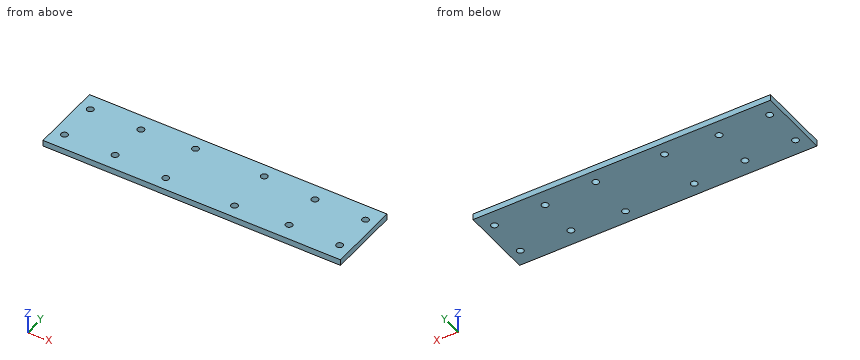
from build123d import *

# Parameters (mm, degrees)
SKETCH_1_W                  = 147
SKETCH_1_H                  = 36
EXTRUDE_1_DEPTH             = 3
HOLE_WIZARD_M4_2_AT_2_COUNT = 2
HOLE_WIZARD_M4_2_AT_2_PITCH = 25


with BuildPart() as part:
    # 草图1 → 凸台-拉伸1 (new body)
    with BuildSketch(Plane.XY):
        Rectangle(SKETCH_1_W, SKETCH_1_H)
    extrude(amount=EXTRUDE_1_DEPTH)

    # 草图3 → M4 螺纹孔的螺纹孔钻头1 (revolve, cut)
    with BuildSketch(Plane(origin=(-17, 11.5, 3), x_dir=(0, -1, 0), z_dir=(1, 0, 0))):
        Polygon((0, 0), (0, 10.991420021), (1.65, 10), (1.65, 0), align=None)
    hole_wizard_m4_1 = revolve(axis=Axis((-17, 11.5, 9.35), (0, 0, -1)), mode=Mode.SUBTRACT)

    # 镜向1: M4 螺纹孔的螺纹孔钻头1 across plane
    add(hole_wizard_m4_1.mirror(Plane.ZX), mode=Mode.SUBTRACT)

    # 镜向2: M4 螺纹孔的螺纹孔钻头1 across plane
    add(hole_wizard_m4_1.mirror(Plane(origin=(0, 0, 0), x_dir=(0, 0, 1), z_dir=(1, 0, 0))), mode=Mode.SUBTRACT)

    # 镜向2 copy 1 sketch → 镜向2 copy 1 (revolve, cut)
    with BuildSketch(Plane(origin=(17, -11.5, 3), x_dir=(0, 1, 0), z_dir=(-1, 0, 0))):
        Polygon((0, 0), (0, 10.991420021), (1.65, 10), (1.65, 0), align=None)
    revolve(axis=Axis((17, -11.5, 9.35), (0, 0, -1)), mode=Mode.SUBTRACT)

    # 草图5 → M4 螺纹孔的螺纹孔钻头2 (revolve, cut)
    with BuildSketch(Plane(origin=(-68, -10, 3), x_dir=(0, -1, 0), z_dir=(1, 0, 0))):
        Polygon((0, 0), (0, 10.991420021), (1.65, 10), (1.65, 0), align=None)
    hole_wizard_m4_2 = revolve(axis=Axis((-68, -10, 9.35), (0, 0, -1)), mode=Mode.SUBTRACT)

    # M4 螺纹孔的螺纹孔钻头2 at 2: M4 螺纹孔的螺纹孔钻头2 ×2
    with Locations(*[(i * HOLE_WIZARD_M4_2_AT_2_PITCH, 0, 0) for i in range(1, HOLE_WIZARD_M4_2_AT_2_COUNT)]):
        add(hole_wizard_m4_2, mode=Mode.SUBTRACT)

    # 镜向3: M4 螺纹孔的螺纹孔钻头2 across plane
    add(hole_wizard_m4_2.mirror(Plane.ZX), mode=Mode.SUBTRACT)

    # 镜向3 copy 1 sketch → 镜向3 copy 1 (revolve, cut)
    with BuildSketch(Plane(origin=(-43, 10, 3), x_dir=(0, 1, 0), z_dir=(1, 0, 0))):
        Polygon((0, 0), (0, -10.991420021), (1.65, -10), (1.65, 0), align=None)
    revolve(axis=Axis((-43, 10, 9.35), (0, 0, 1)), mode=Mode.SUBTRACT)

    # 镜向4: M4 螺纹孔的螺纹孔钻头2 across plane
    add(hole_wizard_m4_2.mirror(Plane(origin=(0, 0, 0), x_dir=(0, 0, 1), z_dir=(1, 0, 0))), mode=Mode.SUBTRACT)

    # 镜向4 copy 1 sketch → 镜向4 copy 1 (revolve, cut)
    with BuildSketch(Plane(origin=(43, -10, 3), x_dir=(0, -1, 0), z_dir=(-1, 0, 0))):
        Polygon((0, 0), (0, -10.991420021), (1.65, -10), (1.65, 0), align=None)
    revolve(axis=Axis((43, -10, 9.35), (0, 0, 1)), mode=Mode.SUBTRACT)

    # 镜向4 copy 2 sketch → 镜向4 copy 2 (revolve, cut)
    with BuildSketch(Plane(origin=(68, 10, 3), x_dir=(0, 1, 0), z_dir=(-1, 0, 0))):
        Polygon((0, 0), (0, 10.991420021), (1.65, 10), (1.65, 0), align=None)
    revolve(axis=Axis((68, 10, 9.35), (0, 0, -1)), mode=Mode.SUBTRACT)

    # 镜向4 copy 3 sketch → 镜向4 copy 3 (revolve, cut)
    with BuildSketch(Plane(origin=(43, 10, 3), x_dir=(0, 1, 0), z_dir=(-1, 0, 0))):
        Polygon((0, 0), (0, 10.991420021), (1.65, 10), (1.65, 0), align=None)
    revolve(axis=Axis((43, 10, 9.35), (0, 0, -1)), mode=Mode.SUBTRACT)


solid = part.part
Check sheet for the modelled part. Datum: model origin and axes. Units: mm. Give positions to 0.01 mm unless a question says otherwise; leave off trailing zeros. Loops run counter-clockwise (first coordinate to the right, second up) from the corner with the lowest first, then second, coordinate; pieces in that order, holes last. Notation, with made-up numbers: M 5,21 L 46,21 A6 cw 46,27 Z; hole C 31.5,47 d10. An arc over 180 degrees is marked long. Answer as a JSON object with one key per item and string values. Group by question number.
Q1. Material ranges on line 1 along Y through (x, z) = (-68, 1.3); line 2 along Y through (x, z) = (-17, 1.1); line 3 along X through (y, z) = (-13, 2.8), recorded low to high. Write a range as [from, to].
Q2. Cross-section at B-B on z = 0.7. Give the number of separate pieces and of enclosed holes in the cut face, then the cut area to 3 significant figures.
Q3. Cross-section at A-A on x = -43. Record the cut outline in (y, z), then the cut area to 3 significant figures.
Q4. Go/stop test with flat-tipped pins: P1, Ø2, axis at x = 17, y = -11.5, coming from the -Z side; P2, Ø5.5, axis at x = 43, y = 10, coming from the +Z side. Record where each tip stops, or that it passes through.
Evaluation:
{
 "1": {"line 1": "y = [-18, -11.65], [-8.35, 8.35], [11.65, 18]", "line 2": "y = [-18, -13.15], [-9.85, 9.85], [13.15, 18]", "line 3": "x = [-73.5, -17.69], [-16.31, 16.31], [17.69, 73.5]"},
 "2": {"separate pieces": "1", "enclosed holes": "12", "area": "5,190 mm2"},
 "3": {"outline": "M -18,0 L -11.65,0 L -11.65,3 L -18,3 Z; M -8.35,0 L 8.35,0 L 8.35,3 L -8.35,3 Z; M 11.65,0 L 18,0 L 18,3 L 11.65,3 Z", "area": "88.2 mm2"},
 "4": {"P1": "passes through", "P2": "stops at z = 3"}
}
